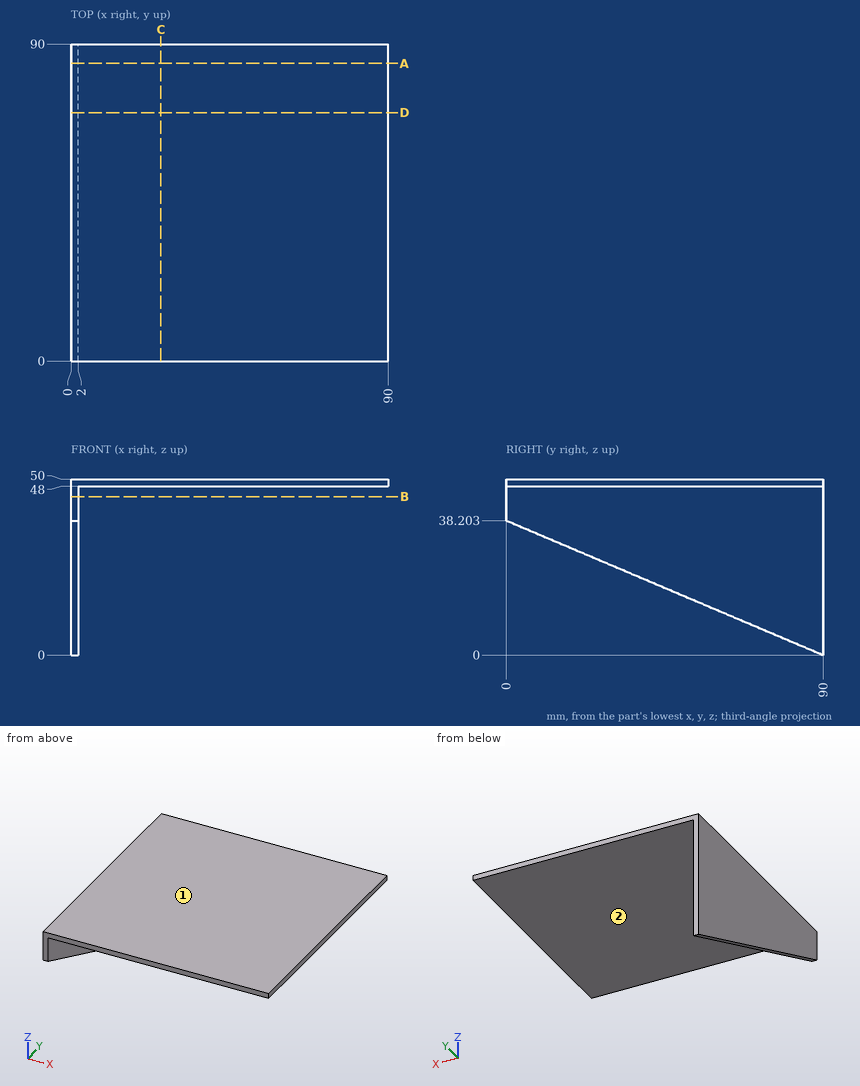
The drawing under review shows one solid part. Ordinate dimensions are in mm from its lowest x, y, z. A direction names the side the tool comes from. Round coordinates to 2 decimals unless told otherwise and drop trailing zeros. Loops run counter-clockwise (first coordinate to the right, second up) from the corner with the lowest first, then second, coordinate; pieces in that order, holes last. Notation, with made-up numbers: (45, 40) - (74, 40) arc R11 ccw to (74, 58) - close; hole circle Ø6 at (68.25, 14.5). An arc over 180 degrees is marked (long way). Use a Markdown table: item, result. Add a question column.
Q1. For probe 1 along X at (y, z) = (76.5, 42); probe 2 along Z at (x, y) = (11, 22.5), list the stretches that pass through material, from the lowest coordinate up.
Q2. Add section D-D (y = 70.5). State the section outline as (x, z) points.
Q3. Add section B-B (z = 45). State the section outline as (x, y) points, plus the area to 3 significant figures.
Q4. Add section A-A (y = 84.5). State the section outline as (x, z) points (1 decimal).
Q5. Add section C-C (x = 25.5). State the section outline as (y, z) points, plus the area to 3 significant figures.
Q6. Machinability: for the marked faces 1 and 2, which of the approach directions +Z, -Z, +X, -X, +Y, -Y give a long, thin tool a straight path to every point of the face, cutting with its end or side? Answer none if there is none.
Q7. Insertion check: pin 1 Ø3 at (x, y) = (80, 80) entering from -Z; pin 2 Ø6 at (y, z) = (34.5, 34) entering from +X. Each pin has a flat end and moves straight along its axis. Give the tip position at first contact, or say it passes through.
Worked answers:
| question | item | result |
|---|---|---|
| 1 | probe 1 | 0 to 2 |
| 1 | probe 2 | 48 to 50 |
| 2 | outline | (0, 8.28) - (2, 8.28) - (2, 48) - (90, 48) - (90, 50) - (0, 50) - close |
| 3 | outline | (0, 0) - (2, 0) - (2, 90) - (0, 90) - close |
| 3 | area | 180 mm² |
| 4 | outline | (0, 2.3) - (2, 2.3) - (2, 48) - (90, 48) - (90, 50) - (0, 50) - close |
| 5 | outline | (0, 48) - (90, 48) - (90, 50) - (0, 50) - close |
| 5 | area | 180 mm² |
| 6 | face 1 | +Z, +X, -X, +Y, -Y |
| 6 | face 2 | -Z, +X, +Y, -Y |
| 7 | pin 1 | z = 48 |
| 7 | pin 2 | x = 2 |
